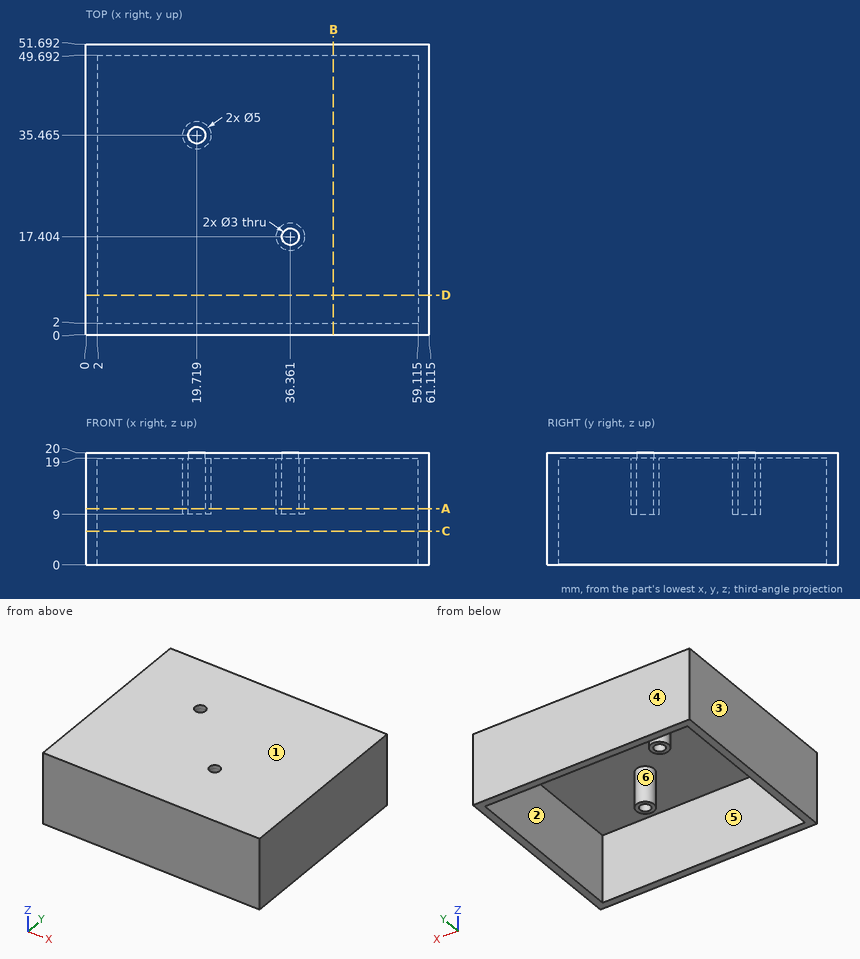
Geometry: see drawing. Coordinates: mm, zero at the bounding-box minimum. A direction names the side the tool comes from. Round coordinates to 2 decimals unless told otherwise and drop trailing zeros. Order: outer loops, then holes, each group sorted by start corner. A loop starts at its lowest first (then second) coordinate and runs counter-clockwise, first axis right, second up. Notation, with made-up numbers: (64, 47.5) -> (95, 47.5) arc R37 cw to (95, 84.5) -> close; hole circle Ø7 at (37, 76). An arc over 180 degrees is marked (long way). Use CSV: the item, a comma, the result in double quotes.
(1) Pull-direction query (X, two-part tool) for the marked faces 3, 4, 5 and 6; classes: +X half, -X half, draft (parallel to the pull), parting line (faces both ways), or undercut.
Report:
face 3,"-X half"
face 4,"draft"
face 5,"undercut"
face 6,"undercut"
(2) Ray query, L1, parallel to Y at x = 22, z = 2.25; L2, parallel to X at y = 13.5, z = 5.25 (1 decimal); L3, parallel to X at y = 15.5, z = 14.25 (1 decimal). Return the intervals inside material, ascending.
Report:
L1,"0 to 2, 49.69 to 51.69"
L2,"0 to 2, 59.1 to 61.1"
L3,"0 to 2, 34.7 to 38, 59.1 to 61.1"
(3) Access query for the marked faces 1 and 2. Directions: +Z, -Z, +X, -X, +Y, -Y. A direction counts if a zero-diameter tool reaches every point of the face in a straight line with its end or side. Return the directions, or none.
Report:
face 1,"+Z, +X, -X, +Y, -Y"
face 2,"-Z"
(4) Section C-C on z = 6. Return the cut outline in (x, y) (1 decimal).
Report:
outline,"(0, 0) -> (61.1, 0) -> (61.1, 51.7) -> (0, 51.7) -> close; hole (2, 2) -> (59.1, 2) -> (59.1, 49.7) -> (2, 49.7) -> close"
(5) Section A-A on z = 10. Return the cut outline in (x, y) (1 decimal).
Report:
outline,"(0, 0) -> (61.1, 0) -> (61.1, 51.7) -> (0, 51.7) -> close; circle Ø5 at (19.7, 35.5); circle Ø5 at (36.4, 17.4); hole (2, 2) -> (59.1, 2) -> (59.1, 49.7) -> (2, 49.7) -> close; hole circle Ø3 at (19.7, 35.5); hole circle Ø3 at (36.4, 17.4)"
(6) Section D-D on y = 7. Return the cut outline in (x, z) (1 decimal), and give its area (3 significant figures).
Report:
outline,"(0, 0) -> (2, 0) -> (2, 19) -> (59.1, 19) -> (59.1, 0) -> (61.1, 0) -> (61.1, 20) -> (0, 20) -> close"
area,"137 mm^2"
(7) Section B-B on x = 44. Return the cut outline in (y, z).
Report:
outline,"(0, 0) -> (2, 0) -> (2, 19) -> (49.69, 19) -> (49.69, 0) -> (51.69, 0) -> (51.69, 20) -> (0, 20) -> close"
(8) First-contact query: pin 1 Ø4 at (x, y) = (19.72, 35.47) entering from -Z. Flat tip, straight axial feed; report the tip coordinate or a pass-through.
Report:
pin 1,"z = 9"
